from build123d import *

# Parameters (mm, degrees)
SKETCH_1_R                        = 2.5
SM_BASE_FLANGE_1_DEPTH            = 5
SM_EDGE_FLANGE_1_STRIP_W          = 26
SM_EDGE_FLANGE_1_STRIP_H          = 5
SM_EDGE_FLANGE_1_STRIP_CUT_DEPTH  = 27.5
SM_EDGE_FLANGE_1_RELIEF_W         = 28.5
SM_EDGE_FLANGE_1_RELIEF_H         = 2.5
SM_EDGE_FLANGE_1_RELIEF_CUT_DEPTH = 5
SM_EDGE_FLANGE_1_DEPTH            = 27.5
EXTRUDE_START                     = -30
SKETCH_9_W                        = 16.25
SKETCH_9_H                        = 16.25
EXTRUDE_1_DEPTH                   = 5
CUT_EXTRUDE_START                 = -30
SKETCH_10_R                       = 3
CUT_EXTRUDE_1_DEPTH               = 5
SKETCH_11_R                       = 2.5
CUT_EXTRUDE_2_DEPTH               = 5


# Sheet-metal steps are written as plain solids
with BuildPart() as part:
    # Sketch 1 → 基体-法兰1 (new body)
    with BuildSketch(Plane(origin=(0, 0, 0), x_dir=(1, 0, 0), z_dir=(0, 1, 0))):
        Polygon((-16.25, 25), (-16.25, 30), (-30, 30), (-30, -30), (-16.25, -30), (-16.25, -25), (16.25, -25), (16.25, -30), (30, -30), (30, 30), (16.25, 30), (16.25, 25), align=None)
        with Locations(Location((-23.75, 23.75, 0), (0, 0, 270))):
            Circle(SKETCH_1_R, mode=Mode.SUBTRACT)
        with Locations(Location((23.75, 23.75, 0), (0, 0, 270))):
            Circle(SKETCH_1_R, mode=Mode.SUBTRACT)
        with Locations(Location((-23.75, -23.75, 0), (0, 0, 270))):
            Circle(SKETCH_1_R, mode=Mode.SUBTRACT)
        with Locations(Location((23.75, -23.75, 0), (0, 0, 270))):
            Circle(SKETCH_1_R, mode=Mode.SUBTRACT)
    extrude(amount=-SM_BASE_FLANGE_1_DEPTH)

    # 边线-法兰1 strip (across the edge) → 边线-法兰1 strip cut (cut)
    with BuildSketch(Plane(origin=(13.75, 0, -25), x_dir=(0, 0, 1), z_dir=(-1, 0, 0))):
        with Locations((-10, -2.5)):
            Rectangle(SM_EDGE_FLANGE_1_STRIP_W, SM_EDGE_FLANGE_1_STRIP_H)
    extrude(amount=SM_EDGE_FLANGE_1_STRIP_CUT_DEPTH, mode=Mode.SUBTRACT)

    # 边线-法兰1 relief (on the sheet) → 边线-法兰1 relief cut (cut)
    with BuildSketch(Plane(origin=(13.75, 0, -22), x_dir=(0, 0, 1), z_dir=(0, 1, 0))):
        with Locations((-11.75, 1.25)):
            Rectangle(SM_EDGE_FLANGE_1_RELIEF_W, SM_EDGE_FLANGE_1_RELIEF_H)
        with Locations((-11.75, -28.75)):
            Rectangle(SM_EDGE_FLANGE_1_RELIEF_W, SM_EDGE_FLANGE_1_RELIEF_H)
    extrude(amount=-SM_EDGE_FLANGE_1_RELIEF_CUT_DEPTH, mode=Mode.SUBTRACT)

    # 边线-法兰1 section (across the edge) → 边线-法兰1 (add)
    with BuildSketch(Plane(origin=(13.75, 0, -25), x_dir=(0, 0, 1), z_dir=(-1, 0, 0))):
        with BuildLine():
            Line((-5, 3), (-5, 70))
            Line((-5, 70), (0, 70))
            Line((0, 70), (0, 3))
            ThreePointArc((0, 3), (0.878679656, 0.878679656), (3, 0))
            Line((3, 0), (3, -5))
            ThreePointArc((3, -5), (-2.656854249, -2.656854249), (-5, 3))
        make_face()
    extrude(amount=SM_EDGE_FLANGE_1_DEPTH)

    # 草图9 → 凸台-拉伸1 (add)
    with BuildSketch(Plane.XY.offset(EXTRUDE_START)):
        with Locations((-21.875, 61.875)):
            Rectangle(SKETCH_9_W, SKETCH_9_H)
        with Locations((21.875, 61.875)):
            Rectangle(SKETCH_9_W, SKETCH_9_H)
        with Locations((-21.875, 18.125)):
            Rectangle(SKETCH_9_W, SKETCH_9_H)
        with Locations((21.875, 18.125)):
            Rectangle(SKETCH_9_W, SKETCH_9_H)
    extrude(amount=EXTRUDE_1_DEPTH)

    # 草图10 → 切除-拉伸1 (cut)
    with BuildSketch(Plane.XY.offset(CUT_EXTRUDE_START)):
        with Locations(Location((0, 50, 0), (0, 0, 90))):
            Circle(SKETCH_10_R)
        with Locations(Location((0, 30, 0), (0, 0, 90))):
            Circle(SKETCH_10_R)
    extrude(amount=CUT_EXTRUDE_1_DEPTH, mode=Mode.SUBTRACT)

    # 草图11 → 切除-拉伸2 (cut)
    with BuildSketch(Plane.XY.offset(CUT_EXTRUDE_START)):
        with Locations(Location((-23.75, 16.25, 0), (0, 0, 90))):
            Circle(SKETCH_11_R)
        with Locations(Location((-23.75, 63.75, 0), (0, 0, 90))):
            Circle(SKETCH_11_R)
        with Locations(Location((23.75, 63.75, 0), (0, 0, 90))):
            Circle(SKETCH_11_R)
        with Locations(Location((23.75, 16.25, 0), (0, 0, 90))):
            Circle(SKETCH_11_R)
    extrude(amount=CUT_EXTRUDE_2_DEPTH, mode=Mode.SUBTRACT)


solid = part.part
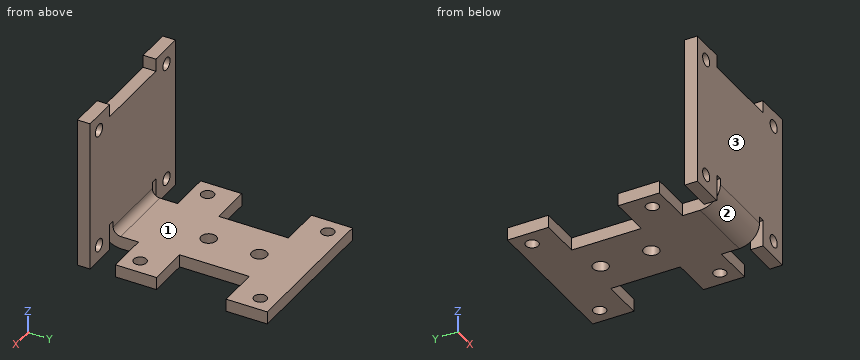
The model under review builds one solid part; all positions refer to its coordinate system, in mm. Face numbers are marked on the shaded views. A direction names the side the tool comes from. Coordinates: 2 decimals unless noted, no trailing zeros. Write each loop counter-clockwise with the first axis right and the second up, starting at its lowest first coordinate (ties: lowest second). Pieces come first, ordered by that corner, then holes. Notation, with made-up numbers: (-20, 53) - (38, 53) arc R32 cw to (38, 85) - close; hole circle Ø9 at (-25.75, 64.5). An arc over 180 degrees is marked (long way). Answer as a JSON object with one key per item and string values. Group by question number.
1. Add section A-A (x = -19). Give the boundary of the cut face in (y, z), plus the area to 4 significant figures.
2. Add section B-B (y = 30). Give the boundary of the cut face in (x, z).
3. Machinability: for the marked faces 1, 2 and 3, which of the approach directions +Z, -Z, +X, -X, +Y, -Y give a long, thin tool a straight path to every point of the face, cutting with its end or side? Answer none if there is none.
4. Add section C-C (z = 23.75). Give the boundary of the cut face in (x, y), plus the area to 3 significant figures.
5. Clearance check with flat-ended pins moving along their axes: pin 1 Ø2 at (x, y) = (-15, -1.5) entering from -Z; pin 2 Ø4 at (x, z) = (-4, 22.5) entering from +Y; pin 3 Ø6 at (x, y) = (-24, 16.5) entering from +Z; pin 4 Ø6 at (x, z) = (23.75, -23.75) entering from +Y. State where each tip first meets the part, or that it passes through.
6. To check wall thickness, follow probe 1 along X at (y, z) = (-3.35, 23.75); probe 2 along Y at (x, z) = (23.75, -27.25); probe 3 along X at (y, z) = (-2.2, -23.75). State the ranges of each line that lie inside material, in increasing order.
7. Add section D-D (z = -23.75). Give the boundary of the cut face in (x, y), plus the area to 3 significant figures.
Findings:
{
 "1": {"outline": "(-5, -30) - (0, -30) - (0, 30) - (-5, 30) - close; (10, -30) - (26.25, -30) - (26.25, -25) - (10, -25) - close; (53.75, -30) - (70, -30) - (70, -25) - (53.75, -25) - close", "area": "462.5 mm²"},
 "2": {"outline": "(-13.75, -30) - (-3, -30) - (-3, -25) - (-13.75, -25) - close; (3, -30) - (13.75, -30) - (13.75, -25) - (3, -25) - close"},
 "3": {"face 1": "+Z, +X, -X, +Y", "face 2": "-Z, -Y", "face 3": "+Z, -Z, +X, -X, -Y"},
 "4": {"outline": "(-30, -5) - (-26.25, -5) - (-26.25, 0) - (-30, 0) - close; (-21.25, -5) - (21.25, -5) - (21.25, 0) - (-21.25, 0) - close; (26.25, -5) - (30, -5) - (30, 0) - (26.25, 0) - close", "area": "250 mm²"},
 "5": {"pin 1": "z = -19.5", "pin 2": "y = 0", "pin 3": "z = -25", "pin 4": "y = 70"},
 "6": {"probe 1": "-30 to -26.25, -21.25 to 21.25, 26.25 to 30", "probe 2": "-5 to 0, 10 to 13.75, 18.75 to 26.25, 53.75 to 61.25, 66.25 to 70", "probe 3": "-30 to -26.25, -21.25 to -16.25, -13.75 to 13.75, 16.25 to 21.25, 26.25 to 30"},
 "7": {"outline": "(-30, -5) - (-26.25, -5) - (-26.25, 0) - (-30, 0) - close; (-21.25, -5) - (-16.25, -5) - (-16.25, 0) - (-21.25, 0) - close; (-13.75, -4.81) - (13.75, -4.81) - (13.75, 0.56) - (-13.75, 0.56) - close; (16.25, -5) - (21.25, -5) - (21.25, 0) - (16.25, 0) - close; (26.25, -5) - (30, -5) - (30, 0) - (26.25, 0) - close", "area": "235 mm²"}
}
